from build123d import *

# Parameters (mm, degrees)
F0_R     = 56
F1_DEPTH = 2
F2_R     = 2
F3_DEPTH = 2
F4_R     = 14
F5_DEPTH = 2


with BuildPart() as f1:
    # F0 (on Top) → F1 (new body)
    with BuildSketch(Plane.XY):
        Circle(F0_R)
    extrude(amount=F1_DEPTH)

    # F2 (on face) → F3 (cut)
    with BuildSketch(Plane.XY.offset(2)):
        Circle(F2_R)
    extrude(amount=-F3_DEPTH, mode=Mode.SUBTRACT)

    # F4 (on face) → F5 (cut)
    with BuildSketch(Plane.XY.offset(2)):
        with Locations((0, 37)):
            Circle(F4_R)
        with Locations((-32.310554, 18.345493)):
            Circle(F4_R)
        with Locations((-32.310554, -18.963521)):
            Circle(F4_R)
        with Locations((0, -37.618028)):
            Circle(F4_R)
        with Locations((32.310554, -18.963521)):
            Circle(F4_R)
        with Locations((32.310554, 18.345493)):
            Circle(F4_R)
    extrude(amount=-F5_DEPTH, mode=Mode.SUBTRACT)


solid = f1.part
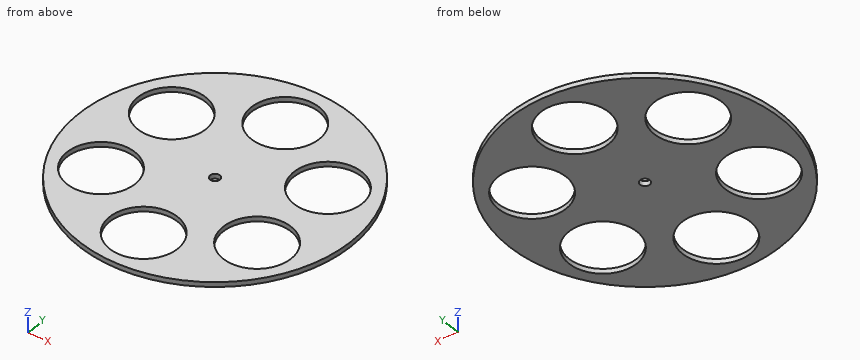
Geometry: final body of the model. Coordinates: model frame, mm. Give positions to 0.01 mm unless a question says otherwise; leave off trailing zeros. Loops run counter-clockwise (first coordinate to the right, second up) from the corner with the lowest first, then second, coordinate; pieces in that order, holes last. Notation, with made-up numbers: (33, 29) -> (82, 29) arc R19 cw to (82, 56) -> close; hole circle Ø6 at (-15, 74.25). An arc over 180 degrees is marked (long way). Put each result on its own line as item: value.
1. Cut plane C-C (x = 24). Return the cut outline in (y, z), plus the area to 3 significant figures.
Taken from the geometry:
outline: (-50.6, 0) -> (-30.23, 0) -> (-30.23, 2) -> (-50.6, 2) -> close; (-7.7, 0) -> (7.08, 0) -> (7.08, 2) -> (-7.7, 2) -> close; (29.61, 0) -> (50.6, 0) -> (50.6, 2) -> (29.61, 2) -> close
area: 112 mm2
2. Ray query, line 1 along Y through (x, z) = (0, 0.95); line 2 along Y through (x, z) = (22.5, 0.75); line 3 along X through (y, z) = (-28.5, 1.75). Return the intervals inside material, ascending. Write a range as [from, to].
Taken from the geometry:
line 1: y = [-56, -51.62], [-23.62, -2], [2, 23], [51, 56]
line 2: y = [-51.28, -28.95], [-8.98, 8.36], [28.33, 51.28]
line 3: x = [-48.21, -42.56], [-22.06, -10.62], [10.62, 22.06], [42.56, 48.21]
3. Cut plane A-A (y = 0). Return the cut outline in (x, z).
Taken from the geometry:
outline: (-56, 0) -> (-2, 0) -> (-2, 2) -> (-56, 2) -> close; (2, 0) -> (56, 0) -> (56, 2) -> (2, 2) -> close
4. Cut plane D-D (y = -28.5). Return the cut outline in (x, z).
Taken from the geometry:
outline: (-48.21, 0) -> (-42.56, 0) -> (-42.56, 2) -> (-48.21, 2) -> close; (-22.06, 0) -> (-10.62, 0) -> (-10.62, 2) -> (-22.06, 2) -> close; (10.62, 0) -> (22.06, 0) -> (22.06, 2) -> (10.62, 2) -> close; (42.56, 0) -> (48.21, 0) -> (48.21, 2) -> (42.56, 2) -> close
5. Pin query (flat end, axial travel): P1, Ø22.5, axis at x = 0, y = -37.62, coming from the -Z side; P2, Ø1, axis at y = 15, z = 1, coming from the -X side. Return the tip coordinate at first contact, or that it passes through.
Taken from the geometry:
P1: passes through
P2: stops at x = -54.09
6. Cut plane B-B (x = 0). Return the cut outline in (y, z).
Taken from the geometry:
outline: (-56, 0) -> (-51.62, 0) -> (-51.62, 2) -> (-56, 2) -> close; (-23.62, 0) -> (-2, 0) -> (-2, 2) -> (-23.62, 2) -> close; (2, 0) -> (23, 0) -> (23, 2) -> (2, 2) -> close; (51, 0) -> (56, 0) -> (56, 2) -> (51, 2) -> close
